```python
from build123d import *

# Parameters (mm, degrees)
SKETCH1_W                = 43
SKETCH1_H                = 45
BOSS_EXTRUDE1_DEPTH      = 5
BOSS_EXTRUDE2_DEPTH      = 22.5
BOSS_EXTRUDE2_DEPTH_BACK = 221.22316262
SKETCH4_W                = 43
SKETCH4_H                = 5
SKETCH5_R                = 2.35
CUT_EXTRUDE2_DEPTH       = 224.06294432
CUT_EXTRUDE3_START       = -13.845143914
CUT_EXTRUDE3_OUTLINE_W   = 12
CUT_EXTRUDE3_OUTLINE_H   = 12
CUT_EXTRUDE3_OUTLINE_R   = 2.35
CUT_EXTRUDE3_DEPTH       = 10.069195574


# Read off the part's stored shape, not the designer's step: Cut-Extrude3
with BuildPart() as part:
    # Sketch1 → Boss-Extrude1 (new body)
    with BuildSketch(Plane(origin=(0, 0, 0), x_dir=(1, 0, 0), z_dir=(0, 1, 0))):
        Rectangle(SKETCH1_W, SKETCH1_H)
    extrude(amount=BOSS_EXTRUDE1_DEPTH)

    # Sketch4 → Boss-Extrude2 (add, two sides: drawn at the far end of the back side and taken through both)
    with BuildSketch(Plane.XY.offset(-BOSS_EXTRUDE2_DEPTH_BACK)):
        Polygon((21.5, 5), (-21.5, 5), (-5, 18.845143914), (5, 18.845143914), align=None)
        with Locations((0, 2.5)):
            Rectangle(SKETCH4_W, SKETCH4_H)
    extrude(amount=BOSS_EXTRUDE2_DEPTH + BOSS_EXTRUDE2_DEPTH_BACK)

    # Sketch5 → Cut-Extrude2 (cut, through all)
    with BuildSketch(Plane.XZ):
        with Locations(Location((15.5, -16.5, 0), (0, 0, 270))):
            Circle(SKETCH5_R)
        with Locations(Location((-15.5, -16.5, 0), (0, 0, 270))):
            Circle(SKETCH5_R)
        with Locations(Location((-15.5, 16.5, 0), (0, 0, 270))):
            Circle(SKETCH5_R)
        with Locations(Location((15.5, 16.5, 0), (0, 0, 270))):
            Circle(SKETCH5_R)
    extrude(amount=-CUT_EXTRUDE2_DEPTH, mode=Mode.SUBTRACT)

    # Cut-Extrude3 outline → Cut-Extrude3 (cut)
    # profile 1 of 4: a face of its own
    with BuildSketch(Plane(origin=(0, 18.845143914, 0), x_dir=(1, 0, 0), z_dir=(0, 1, 0)).offset(CUT_EXTRUDE3_START)):
        with Locations((-15.5, 16.5)):
            Rectangle(CUT_EXTRUDE3_OUTLINE_W, CUT_EXTRUDE3_OUTLINE_H)
        with Locations((-15.5, 16.5)):
            Circle(CUT_EXTRUDE3_OUTLINE_R, mode=Mode.SUBTRACT)
    # profile 2 of 4: a face of its own
    with BuildSketch(Plane(origin=(0, 18.845143914, 0), x_dir=(1, 0, 0), z_dir=(0, 1, 0)).offset(CUT_EXTRUDE3_START)):
        with Locations((-15.5, -16.5)):
            Rectangle(CUT_EXTRUDE3_OUTLINE_W, CUT_EXTRUDE3_OUTLINE_H)
        with Locations((-15.5, -16.5)):
            Circle(CUT_EXTRUDE3_OUTLINE_R, mode=Mode.SUBTRACT)
    # profile 3 of 4: a face of its own
    with BuildSketch(Plane(origin=(0, 18.845143914, 0), x_dir=(1, 0, 0), z_dir=(0, 1, 0)).offset(CUT_EXTRUDE3_START)):
        with Locations((15.5, 16.5)):
            Rectangle(CUT_EXTRUDE3_OUTLINE_W, CUT_EXTRUDE3_OUTLINE_H)
        with Locations((15.5, 16.5)):
            Circle(CUT_EXTRUDE3_OUTLINE_R, mode=Mode.SUBTRACT)
    # profile 4 of 4: a face of its own
    with BuildSketch(Plane(origin=(0, 18.845143914, 0), x_dir=(1, 0, 0), z_dir=(0, 1, 0)).offset(CUT_EXTRUDE3_START)):
        with Locations((15.5, -16.5)):
            Rectangle(CUT_EXTRUDE3_OUTLINE_W, CUT_EXTRUDE3_OUTLINE_H)
        with Locations((15.5, -16.5)):
            Circle(CUT_EXTRUDE3_OUTLINE_R, mode=Mode.SUBTRACT)
    extrude(amount=CUT_EXTRUDE3_DEPTH, mode=Mode.SUBTRACT)


solid = part.part
```
Build history of the part. All positions in model axes, mm. A direction names the side the tool comes from. Give positions to 0.01 mm unless a question says otherwise; leave off trailing zeros. Loops run counter-clockwise (first coordinate to the right, second up) from the corner with the lowest first, then second, coordinate; pieces in that order, holes last. Notation, with made-up numbers: (12, 40.25) - (29, 40.25) arc R34 ccw to (29, 71.25) - close; hole circle Ø5 at (80, 32.5). An arc over 180 degrees is marked (long way). Use a Markdown table: item, result.
(1) Which spindle directions (+Z, -Z, +X, -X, +Y, -Y) get a long thin tool onto all of the face, cutting with end or side? Do faces 1 (the face through (-13, 8, -22.5)), 2 (the face through (14, 9, -22.5)), 3 (the face through (18, 5, 16)). Say none if no direction does.
Taken from the geometry:
| item | result |
|---|---|
| face 1 | -X, +Y |
| face 2 | +X, +Y |
| face 3 | +Z, +X, +Y |
(2) Band-saw the part on B-B (x = -15.5). Give the cut face in (y, z), and give its area (3 significant figures).
Taken from the geometry:
| item | result |
|---|---|
| outline | (0, -221.22) - (10.03, -221.22) - (10.03, -22.5) - (5, -22.5) - (5, -18.85) - (0, -18.85) - close; (0, -14.15) - (5, -14.15) - (5, -10.5) - (10.03, -10.5) - (10.03, 10.5) - (5, 10.5) - (5, 14.15) - (0, 14.15) - close; (0, 18.85) - (5, 18.85) - (5, 22.5) - (0, 22.5) - close |
| area | 2,280 mm2 |
(3) Band-saw the part on A-A (z = -16.5). Give the cut face in (x, y), and give its area (3 significant figures).
Taken from the geometry:
| item | result |
|---|---|
| outline | (-21.5, 0) - (-17.85, 0) - (-17.85, 5) - (-21.5, 5) - close; (-13.15, 0) - (13.15, 0) - (13.15, 5) - (9.5, 5) - (9.5, 15.07) - (5, 18.85) - (-5, 18.85) - (-9.5, 15.07) - (-9.5, 5) - (-13.15, 5) - close; (17.85, 0) - (21.5, 0) - (21.5, 5) - (17.85, 5) - close |
| area | 414 mm2 |
(4) Wall check: line 1 along X through (y, z) = (1.4, -16.5); line 2 along Z through (x, y) = (15.5, 2.8); line 3 along Z through (x, y) = (10.5, 8). Give the ranges that are in metal, low to high.
Taken from the geometry:
| item | result |
|---|---|
| line 1 | -21.5 to -17.85, -13.15 to 13.15, 17.85 to 21.5 |
| line 2 | -221.22 to -18.85, -14.15 to 14.15, 18.85 to 22.5 |
| line 3 | -221.22 to -22.5, -10.5 to 10.5 |
(5) Band-saw the part on C-C (z = -50). Give the cut face in (x, y).
Taken from the geometry:
| item | result |
|---|---|
| outline | (-21.5, 0) - (21.5, 0) - (21.5, 5) - (5, 18.85) - (-5, 18.85) - (-21.5, 5) - close |
(6) Drop flat-ended pins along their axis: pin 1 Ø5 at (y, z) = (9, -17) entering from +X; pin 2 Ø6 at (x, z) = (15.5, 17) entering from +Y; pin 3 Ø1 at (y, z) = (13, -68) entering from +X. Give the stop position or say it passes through.
Taken from the geometry:
| item | result |
|---|---|
| pin 1 | x = 9.5 |
| pin 2 | y = 5 |
| pin 3 | x = 12.56 |
(7) Pull direction Z, two halves, no side cores. Call faces 4 (the face through (14.07, 2.465, 18.365)), 5 (the face through (-9.5, 10, 17)), 6 (the face through (14, 9, 10.5)), 7 (the face through (0, 7, -221.223)): +Z half, -Z half, draft (parallel to the pull), parting line (faces both ways), or undercut.
Taken from the geometry:
| item | result |
|---|---|
| face 4 | undercut |
| face 5 | draft |
| face 6 | +Z half |
| face 7 | -Z half |
